Part model, mm, in its own coordinate system. Face numbers are marked on the shaded views. A direction names the side the tool comes from. Round coordinates to 2 decimals unless told otherwise and drop trailing zeros. Write each loop counter-clockwise with the first axis right and the second up, starting at its lowest first coordinate (ties: lowest second). Pieces come first, ordered by that corner, then holes.
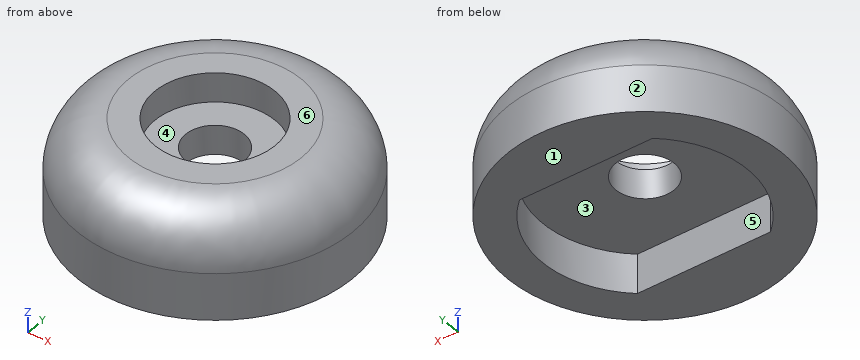
Autodesk Inventor part; units mm, degrees
ref_plane "Work Plane1" through (-12.875, -12.875, -1.15) normal (0, 0, 1) x (1, 0, 0)
ref_plane "YZ Plane" through (0, 0, 0) normal (1, 0, 0) x (0, 1, 0)
ref_plane "XZ Plane" through (0, 0, 0) normal (0, 1, 0) x (-1, 0, 0)
sketch "Sketch1" plane through (0, 0, 0) normal (0, 0, 1) x (1, 0, 0)
  circle A0 centre (0, 0) radius 4.7
  circle A1 centre (0, 0) radius 1
  arc A2 (-2.2864, 2.65) -> (-2.2864, -2.65) centre (0, 0) ccw
  line L0 (-2.2864, -2.65) -> (2.2864, -2.65)
  line L1 (2.2864, 2.65) -> (-2.2864, 2.65)
  arc A3 (2.2864, -2.65) -> (2.2864, 2.65) centre (0, 0) ccw
ref_plane "Work Plane1" through (-12.875, -12.875, -1.15) normal (0, 0, 1) x (1, 0, 0)
extrude "Extrusion1" add sketch "Sketch1" along normal blind 0.2 and the other way blind 1.15 contours A0
sketch "Sketch2" plane through (0, 0, 0.2) normal (0, 0, 1) x (1, 0, 0)
  circle A0 centre (0, 0) radius 4.7
  circle A1 centre (0, 0) radius 1
extrude "Extrusion2" add sketch "Sketch2" along normal blind 2
fillet "Fillet1" radius 1.75 1 edges at (-4.7, 0, 2.2)
sketch "Sketch3" plane through (0, 0, 2.2) normal (0, 0, 1) x (1, 0, 0)
  circle A0 centre (0, 0) radius 2.05
  circle A1 centre (0, 0) radius 1
  point P0 (0, 0)
  dimension "d7" = 4.1
extrude "Extrusion3" cut sketch "Sketch3" against normal blind 1 contours A0 | A1
properties part number "TTencodercap"
Q1. Cut at B-B on y = 0. Write the cut outline in (x, z).
Values follow:
outline: (-4.7, -1.15) - (-3.5, -1.15) - (-3.5, 0.2) - (-1, 0.2) - (-1, 1.2) - (-2.05, 1.2) - (-2.05, 2.2) - (-2.95, 2.2) arc R1.75 ccw to (-4.7, 0.45) - close; (1, 0.2) - (3.5, 0.2) - (3.5, -1.15) - (4.7, -1.15) - (4.7, 0.45) arc R1.75 ccw to (2.95, 2.2) - (2.05, 2.2) - (2.05, 1.2) - (1, 1.2) - close
Q2. Cut at C-C on z = -0.4. Write the cut outline in (x, y), plus the area to 3 significant figures.
Values follow:
outline: circle Ø9.4 at (0, 0); hole (-2.29, -2.65) - (2.29, -2.65) arc R3.5 ccw to (2.29, 2.65) - (-2.29, 2.65) arc R3.5 ccw to start
area: 36.2 mm2
Q3. Drop flat-ended pins along their axis: pin 1 (3.5 mm diameter, centred on x = 0, y = 0, fed in from -Z); pin 2 (1.5 mm diameter, centred on x = 1, z = 0, fed in from -Y); pin 3 (1.5 mm diameter, centred on x = -4, z = 0.5, fed in from -Y). Give the stop position or say it passes through.
Values follow:
pin 1: stops at z = 0.2
pin 2: stops at y = -4.69
pin 3: stops at y = -3.39
Q4. Cut at D-D on z = 1.75. Write the cut outline in (x, y).
Values follow:
outline: circle Ø8.24 at (0, 0); hole circle Ø4.1 at (0, 0)
Q5. Which spindle directions (+Z, -Z, +X, -X, +Y, -Y) get a long thin tool onto all of the face, cutting with end or side? Do the marked faces 4, 5 and 6. Say none if no direction does.
Values follow:
face 4: +Z
face 5: -Z
face 6: +Z, +X, -X, +Y, -Y
Q6. Wall check: L1, parallel to Z at x = -0.25, y = -1; L2, parallel to Y at x = 0, z = 2.05; L3, parallel to Z at x = 1.5, y = 2. Give the ranges that are in metal, low to high.
Values follow:
L1: z = 0.2 to 1.2
L2: y = -3.66 to -2.05, 2.05 to 3.66
L3: z = 0.2 to 2.2
Q7. Cut at A-A on x = 0. Write the cut outline in (y, z), plus the area to 3 significant figures.
Values follow:
outline: (-4.7, -1.15) - (-2.65, -1.15) - (-2.65, 0.2) - (-1, 0.2) - (-1, 1.2) - (-2.05, 1.2) - (-2.05, 2.2) - (-2.95, 2.2) arc R1.75 ccw to (-4.7, 0.45) - close; (1, 0.2) - (2.65, 0.2) - (2.65, -1.15) - (4.7, -1.15) - (4.7, 0.45) arc R1.75 ccw to (2.95, 2.2) - (2.05, 2.2) - (2.05, 1.2) - (1, 1.2) - close
area: 16.9 mm2
Q8. Mould opens along Y. For the marked faces 1, 2 and 3 say: +Y half, -Y half, draft (parallel to the pull), parting line (faces both ways), or undercut.
Values follow:
face 1: draft
face 2: parting line
face 3: undercut
